from build123d import *

# Parameters (mm, degrees)
SKETCH1_R           = 12.5
BOSS_EXTRUDE1_DEPTH = 7.5
SKETCH4_W           = 4
SKETCH4_H           = 27.5
BOSS_EXTRUDE3_DEPTH = 15
CIRPATTERN7_COUNT   = 6
SKETCH7_R           = 1.45
CUT_EXTRUDE2_DEPTH  = 17
CIRPATTERN9_COUNT   = 6
CUT_EXTRUDE3_REACH  = 43.398
SKETCH8_W           = 12.15
SKETCH8_H           = 12.15
SKETCH9_R           = 1.45
CUT_EXTRUDE4_DEPTH  = 10


with BuildPart() as part:
    # Sketch1 → Boss-Extrude1 (new, symmetric)
    with BuildSketch(Plane.XY):
        Circle(SKETCH1_R)
    extrude(amount=BOSS_EXTRUDE1_DEPTH, both=True)

    # Sketch4 → Boss-Extrude3 (add)
    with BuildSketch(Plane.XY.offset(7.5)):
        with Locations((-4.5, 13.75)):
            Rectangle(SKETCH4_W, SKETCH4_H)
        with Locations((4.5, 13.75)):
            Rectangle(SKETCH4_W, SKETCH4_H)
    boss_extrude3 = extrude(amount=-BOSS_EXTRUDE3_DEPTH)

    # CirPattern7: Boss-Extrude3 ×6 about axis
    cirpattern7_axis = Axis((0, 0, 0), (0, 0, 1))
    for i in range(1, CIRPATTERN7_COUNT):
        add(boss_extrude3.rotate(cirpattern7_axis, i * 360 / CIRPATTERN7_COUNT))

    # Sketch7 → Cut-Extrude2 (cut)
    with BuildSketch(Plane.ZY.offset(6.5)):
        with Locations((0, 20)):
            Circle(SKETCH7_R)
        with Locations((40, 20)):
            Circle(SKETCH7_R)
        with Locations((80, 20)):
            Circle(SKETCH7_R)
        with Locations((120, 20)):
            Circle(SKETCH7_R)
        with Locations((160, 20)):
            Circle(SKETCH7_R)
    cut_extrude2 = extrude(amount=-CUT_EXTRUDE2_DEPTH, mode=Mode.SUBTRACT)

    # CirPattern9: Cut-Extrude2 ×6 about axis
    cirpattern9_axis = Axis((0, 0, 0), (0, 0, 1))
    for i in range(1, CIRPATTERN9_COUNT):
        add(cut_extrude2.rotate(cirpattern9_axis, i * 360 / CIRPATTERN9_COUNT), mode=Mode.SUBTRACT)

    # Sketch8 → Cut-Extrude3 (cut, up to next)
    with BuildSketch(Plane.XY.offset(7.5), mode=Mode.PRIVATE) as cut_extrude3_sk1:
        Rectangle(SKETCH8_W, SKETCH8_H)
    cut_extrude3_tool1 = extrude(cut_extrude3_sk1.sketch, amount=-CUT_EXTRUDE3_REACH, mode=Mode.PRIVATE) & part.part
    add(cut_extrude3_tool1.solids().sort_by_distance((0, 0, 7.5))[0], mode=Mode.SUBTRACT)

    # Sketch9 → Cut-Extrude4 (cut)
    with BuildSketch(Plane.XY.offset(7.5)):
        with Locations((9.2875, 0)):
            Circle(SKETCH9_R)
        with Locations((0, -9.2875)):
            Circle(SKETCH9_R)
        with Locations((-9.2875, 0)):
            Circle(SKETCH9_R)
        with Locations((0, 9.2875)):
            Circle(SKETCH9_R)
    extrude(amount=-CUT_EXTRUDE4_DEPTH, mode=Mode.SUBTRACT)


solid = part.part
Can you work these out from the model? Positions are in its coordinate system, mm. A direction names the side the tool comes from. Give positions to 0.01 mm unless a question says otherwise; leave off trailing zeros. Order: outer loops, then holes, each group sorted by start corner. A loop starts at its lowest first (then second) coordinate and runs counter-clockwise, first axis right, second up. Notation, with made-up numbers: M 48.5,19 L 89.5,19 A13 ccw 89.5,43 Z; hole C 54,-21 d2. An arc over 180 degrees is marked long. Use one line per item in the form item = value. Start each with the question number.
Item 1: We'd pull the mould along X, two halves only. Please class faces 5 (the flat face through (-21.58, 17.62, 0.11)), 6 (the flat face through (-2.5, 20, 2)), 7 (the flat face through (1.2, -6.4, 7.5)): +X half, -X half, draft (parallel to the pull), parting line (faces both ways), or undercut.
Item 2: For faces 1 (the flat face through (6.5, -19, 2)), 2 (the flat face through (-15.87, 12.05, 1.77)), 3 (the flat face through (-19.93, -4, 1.77)), 4 (the flat face through (-9, 0, -2.5)), which set-ups out of +Z, -Z, +X, -X, +Y, -Y let a thin tool reach every point of the face, with its end or its side?
Item 3: If we section it at A-A (x = 0): Write out the boundary of the cut face in (y, z) (1 decimal), then the cut area to 3 significant figures.
Item 4: If we section it at B-B (z = 0.5): State how many separate pieces and enclosed holes the cut face has, then the cut area to 3 significant figures.
Item 5: Will these pins go through, and if not, where does the flat tip stop? pin 1 Ø1.5 at (y, z) = (20, -5.5) entering from -X; pin 2 Ø8 at (y, z) = (1.5, -5.5) entering from -X; pin 3 Ø7.5 at (y, z) = (-22, -3) entering from -X; pin 4 Ø3 at (x, y) = (-9, 0) entering from +Z.
Item 6: If I drill on line 1 along Y through (x, z) = (0, 4) (1 decimal); line 2 along X through (y, z) = (-25, -4.25); line 3 along Y through (x, z) = (-4.15, 0) (3 decimals), over which ranges is the centre line in solid material (lowest first)?
Outcome:
q1.face_5 = -X half
q1.face_6 = undercut
q1.face_7 = draft
q2.face_1 = +Z, -Z, -Y
q2.face_2 = +Z, -Z
q2.face_3 = +Z, -Z, -X
q2.face_4 = +Z
q3.outline = M -12.5,-7.5 L -6.1,-7.5 L -6.1,7.5 L -7.8,7.5 L -7.8,-2.5 L -10.7,-2.5 L -10.7,7.5 L -12.5,7.5 Z; M 6.1,-7.5 L 12.5,-7.5 L 12.5,7.5 L 10.7,7.5 L 10.7,-2.5 L 7.8,-2.5 L 7.8,7.5 L 6.1,7.5 Z
q3.area = 135 mm2
q4.separate_pieces = 13
q4.enclosed_holes = 5
q4.area = 949 mm2
q5.pin_1 = -20.64
q5.pin_2 = -22.53
q5.pin_3 = -21.22
q5.pin_4 = 7.5
q6.line_1 = -12.5 to -10.7, -7.8 to -6.1, 6.1 to 7.8, 10.7 to 12.5
q6.line_2 = -6.5 to -2.5, 2.5 to 6.5
q6.line_3 = -27.5 to -21.45, -18.55 to -6.075, 6.075 to 18.55, 21.45 to 27.5
